Source: CAD feature listing. Evaluate the final solid. Frame: model axes, mm. Face numbers are marked on the shaded views. Coordinates: 2 decimals unless noted, no trailing zeros. Write each loop counter-clockwise with the first axis right and the second up, starting at its lowest first coordinate (ties: lowest second). Pieces come first, ordered by that corner, then holes. Notation, with made-up numbers: (56, -26) - (93, -26) arc R24 ccw to (93, 10) - close; hole circle Ø1 at (89.5, 48.25). An arc over 180 degrees is marked (long way). One line per item, written item: value.
from build123d import *

# Parameters (mm, degrees)
SKETCH1_W           = 2
SKETCH1_H           = 40
SKETCH1_W_2         = 3
SKETCH1_H_2         = 10
BOSS_EXTRUDE1_DEPTH = 2.5
FILLET1_R           = 0.5
FILLET2_R           = 1
FILLET3_R           = 1
FILLET4_R           = 2


with BuildPart() as part:
    # Sketch1 → Boss-Extrude1 (new, symmetric)
    with BuildSketch(Plane.XY):
        with BuildLine():
            Line((-18.6, 166.579989158), (-18.6, 182.956591985))
            Line((-18.6, 182.956591985), (-21.85, 182.956591985))
            Line((-21.85, 182.956591985), (-21.85, 183.956591985))
            Line((-21.85, 183.956591985), (-18.6, 183.956591985))
            Line((-18.6, 183.956591985), (-18.6, 192.579989158))
            Line((-18.6, 192.579989158), (-16.6, 192.579989158))
            Line((-16.6, 192.579989158), (-16.6, 196.474649456))
            Line((-16.6, 196.474649456), (-29.6, 196.474649456))
            Line((-29.6, 196.474649456), (-29.6, 192.579989158))
            Line((-29.6, 192.579989158), (-27.6, 192.579989158))
            Line((-27.6, 192.579989158), (-27.6, 167.706591985))
            Line((-27.6, 167.706591985), (-47.6, 164.206591985))
            Line((-47.6, 164.206591985), (-47.6, 159.206591985))
            Line((-47.6, 159.206591985), (-27.6, 155.706591985))
            Line((-27.6, 155.706591985), (-27.6, 129.579989158))
            Line((-27.6, 129.579989158), (-29.6, 129.579989158))
            Line((-29.6, 129.579989158), (-29.6, 125.685328859))
            Line((-29.6, 125.685328859), (-27.6, 125.685328859))
            Line((-27.6, 125.685328859), (-27.6, 94.474649456))
            Line((-27.6, 94.474649456), (-18.6, 94.474649456))
            Line((-18.6, 94.474649456), (-18.6, 125.685328859))
            Line((-18.6, 125.685328859), (-16.6, 125.685328859))
            Line((-16.6, 125.685328859), (-16.6, 129.579989158))
            Line((-16.6, 129.579989158), (-18.6, 129.579989158))
            Line((-18.6, 129.579989158), (-18.6, 139.456591985))
            Line((-18.6, 139.456591985), (-21.85, 139.456591985))
            Line((-21.85, 139.456591985), (-21.85, 140.456591985))
            Line((-21.85, 140.456591985), (-18.6, 140.456591985))
            Line((-18.6, 140.456591985), (-18.6, 156.833194813))
            ThreePointArc((-18.6, 156.833194813), (-16.1, 161.706591985), (-18.6, 166.579989158))
        make_face()
        with Locations((-20.85, 161.706591985)):
            Rectangle(SKETCH1_W, SKETCH1_H, mode=Mode.SUBTRACT)
        with Locations((-22.6, 109.474649456)):
            Rectangle(SKETCH1_W_2, SKETCH1_H_2, mode=Mode.SUBTRACT)
    extrude(amount=BOSS_EXTRUDE1_DEPTH, both=True)

    # Fillet1
    fillet1_edges = [part.edges().sort_by_distance(p)[0] for p in [
        (-21.85, 183.956591985, 0),
        (-21.85, 182.956591985, 0),
        (-21.85, 140.456591985, 0),
        (-21.85, 139.456591985, 0),
        (-21.85, 181.706591985, 0),
        (-21.85, 141.706591985, 0),
        (-19.85, 141.706591985, 0),
        (-19.85, 181.706591985, 0),
    ]]
    fillet(fillet1_edges, radius=FILLET1_R - 0.0001)  # a hair under: the kernel refuses the full size

    # Fillet2
    fillet2_edges = [part.edges().sort_by_distance(p)[0] for p in [
        (-18.6, 182.956591985, 0),
        (-18.6, 140.456591985, 0),
    ]]
    fillet(fillet2_edges, radius=FILLET2_R)

    # Fillet3
    fillet3_edges = [part.edges().sort_by_distance(p)[0] for p in [
        (-18.6, 166.579989158, 0),
        (-18.6, 156.833194813, 0),
    ]]
    fillet(fillet3_edges, radius=FILLET3_R)

    # Fillet4
    fillet4_edges = [part.edges().sort_by_distance(p)[0] for p in [
        (-27.6, 155.706591985, 0),
        (-47.6, 159.206591985, 0),
        (-47.6, 164.206591985, 0),
        (-27.6, 167.706591985, 0),
    ]]
    fillet(fillet4_edges, radius=FILLET4_R)


solid = part.part
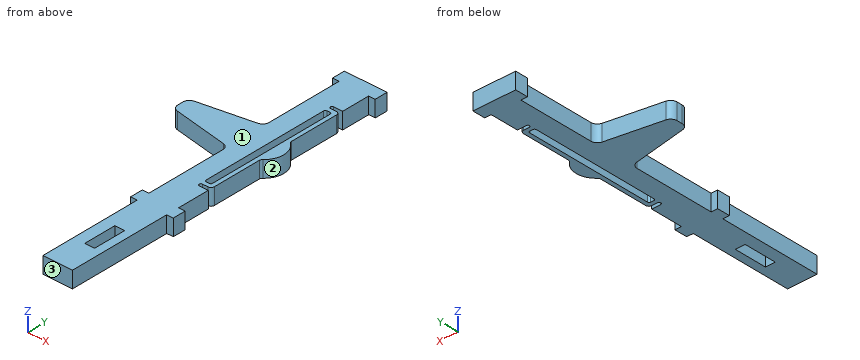
1) Section query C-C on x = -44. Output: boundary loops of the cut face in (y, z), then the cut area to 3 significant figures.
Values found:
outline: (158.58, -2.5) - (164.84, -2.5) - (164.84, 2.5) - (158.58, 2.5) - close
area: 31.3 mm2
2) Section query B-B on y = 103. Output: boundary loops of the cut face in (x, z), then the cut area to 3 significant figures.
Values found:
outline: (-27.6, -2.5) - (-18.6, -2.5) - (-18.6, 2.5) - (-27.6, 2.5) - close
area: 45.0 mm2
3) Material intervals for line 1 (X direction, y = 151.5, z = 0.15); line 2 (X direction, y = 114, z = -1.3); line 3 (Y direction, x = -19, z = -1.85), sorted ascending.
Values found:
line 1: -27.6 to -21.85, -19.85 to -18.6
line 2: -27.6 to -24.1, -21.1 to -18.6
line 3: 94.47 to 139.46, 140.66 to 182.76, 183.96 to 196.47
4) Draft query along Y for the marked faces 1, 2 and 3. Return one class per face: released by +Y, released by -Y, zero draft, split by the parting line, or undercut.
Values found:
face 1: zero draft
face 2: undercut
face 3: released by -Y
5) Contact query for flat-ended pins moving along their axis: P1, Ø2, axis at x = -29, z = 0.5, coming from the -Y side; P2, Ø1.5, axis at y = 145.5, z = 1, coming from the +X side; P3, Ø2, axis at y = 163, z = -1.5, coming from the +X side. Output: stop coordinate, or through.
Values found:
P1: y = 125.69
P2: x = -18.6
P3: x = -16.11
6) Section query A-A on z = 1.2. State how many separate pieces and enclosed holes the cut face has, then the cut area to 3 significant figures.
Values found:
separate pieces: 1
enclosed holes: 2
area: 1,020 mm2
